Source: three-view drawing plus pictorial views. Frame: mm from the lowest corner of the part. Round coordinates to 2 decimals unless told otherwise and drop trailing zeros. Loops run counter-clockwise (first coordinate to the right, second up) from the corner with the lowest first, then second, coordinate; pieces in that order, holes last. Notation, with made-up numbers: M 12.5,39 L 55.5,39 A25 cw 55.5,68 Z; hole C -19,-30.75 d8. An arc over 180 degrees is marked long. Write each question's results on one line, items separated by ' | '.
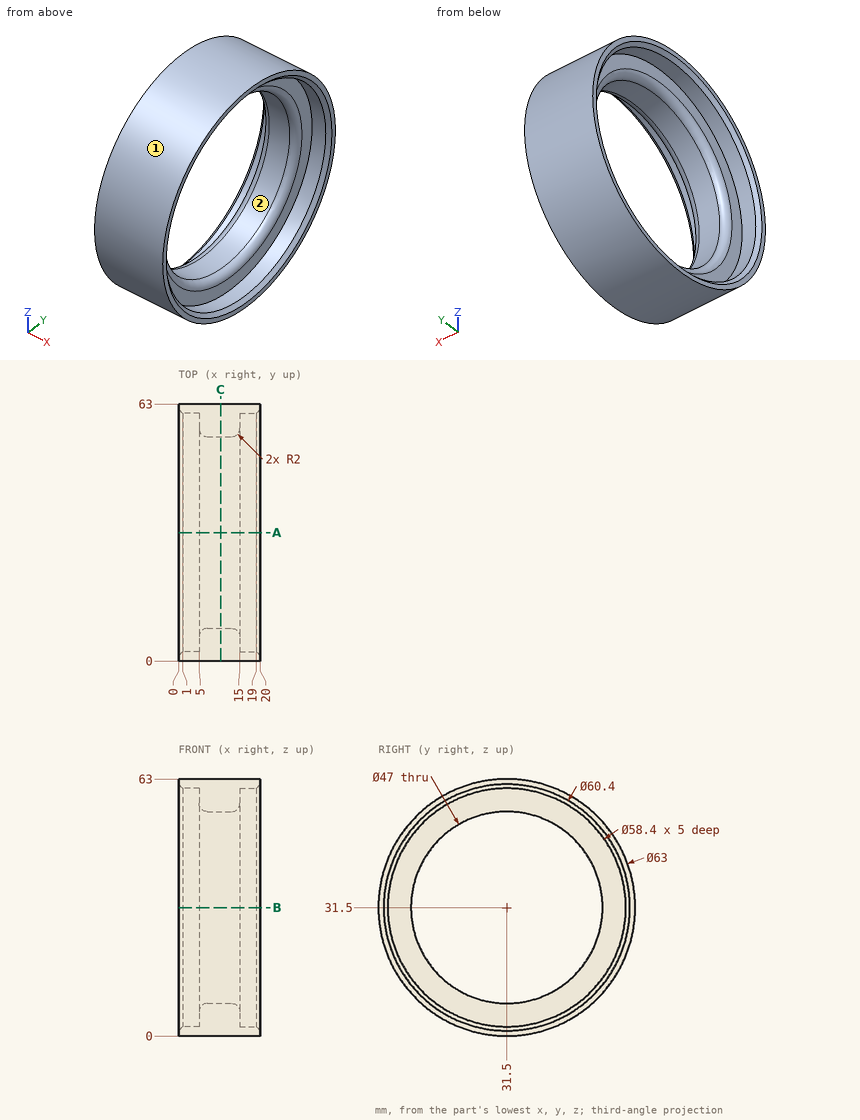
1. Ray query, probe 1 along Z at (x, y) = (16.1, 31.5); probe 2 along X at (y, z) = (44, 53.5); probe 3 along Z at (x, y) = (10.45, 31.5). Return the intervals inside material, ascending.
Answer key:
probe 1: z = 0 to 2.3, 60.7 to 63 | probe 2: x = 5.01 to 14.99 | probe 3: z = 0 to 8, 55 to 63
2. Draft query along Z for the marked faces 1 and 2. Return one class per face: pulls with the +Z half, pulls with the -Z half, needs draft (parallel to the pull), parting line crosses it, or undercut.
Answer key:
face 1: parting line crosses it | face 2: undercut
3. Section C-C (x = 10.25). Output: boundary loops of the cut face in (y, z), then the cut area to 3 significant figures.
Answer key:
outline: C 31.5,31.5 d63; hole C 31.5,31.5 d47 | area: 1,380 mm²
4. Section A-A (y = 31.5). Output: boundary loops of the cut face in (x, z), then the cut area to 3 significant figures.
Answer key:
outline: M 0,0 L 20,0 L 20,1.3 L 19,2.3 L 15,2.3 L 15,6 A2 ccw 13,8 L 7,8 A2 ccw 5,6 L 5,2.3 L 1,2.3 L 0,1.3 Z; M 0,61.7 L 1,60.7 L 5,60.7 L 5,57 A2 ccw 7,55 L 13,55 A2 ccw 15,57 L 15,60.7 L 19,60.7 L 20,61.7 L 20,63 L 0,63 Z | area: 201 mm²
5. Pin query (flat end, axial travel): P1, Ø4, axis at x = 4.5, y = 31.5, coming from the +Z side; P2, Ø8, axis at x = 3, y = 34.5, coming from the -Z side; P3, Ø12, axis at x = 8.5, z = 53.5, coming from the +Y side. Return the tip coordinate at first contact, or that it passes through.
Answer key:
P1: stops at z = 63 | P2: stops at z = 0 | P3: stops at y = 58.63
